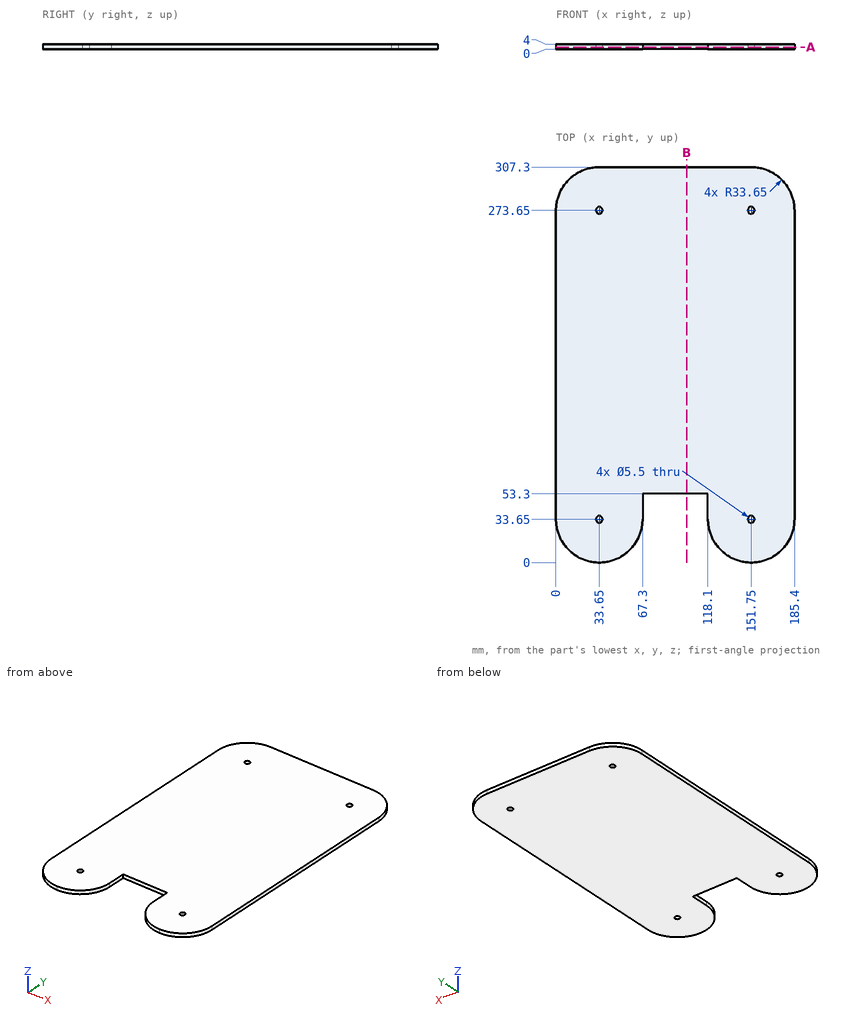
Verification items for this drawing (mm, ordinates from the low corner). Give positions to 0.01 mm unless a question says otherwise; leave off trailing zeros. Write each loop counter-clockwise with the first axis right and the second up, starting at its lowest first coordinate (ties: lowest second). Pieces come first, ordered by that corner, then holes.
1) Gauge pin test, flat ends, axial feed: pin 1 (1 mm diameter, centred on x = 28.5, z = 1.5, fed in from -Y); pin 2 (2 mm diameter, centred on y = 47.5, z = 2.5, fed in from -X); pin 3 (1 mm diameter, centred on x = 141.5, z = 2.5, fed in from -Y). Record the tip position at first contact, or that the pin passes through.
2) Section check A-A, the plane z = 1.65. Record the boundary of the cut face in (x, y), and give its area (3 significant figures).
3) Section check B-B, the plane x = 101.5. Record the boundary of the cut face in (y, z).
4) Material ranges on L1, parallel to Y at x = 151.75, z = 2.65; L2, parallel to X at y = 20, z = 3.5; L3, parallel to X at y = 21, z = 2, recorded low to high.
Computed:
1. pin 1: stops at y = 0.32
1. pin 2: stops at x = 0
1. pin 3: stops at y = 1.44
2. outline: (0, 33.65) arc R33.65 ccw to (67.3, 33.65) - (67.3, 53.3) - (118.1, 53.3) - (118.1, 33.65) arc R33.65 ccw to (185.4, 33.65) - (185.4, 273.65) arc R33.65 ccw to (151.75, 307.3) - (33.65, 307.3) arc R33.65 ccw to (0, 273.65) - close; hole circle Ø5.5 at (33.65, 33.65); hole circle Ø5.5 at (33.65, 273.65); hole circle Ø5.5 at (151.75, 33.65); hole circle Ø5.5 at (151.75, 273.65)
2. area: 52,700 mm2
3. outline: (53.3, 0) - (307.3, 0) - (307.3, 4) - (53.3, 4) - close
4. L1: y = 0 to 30.9, 36.4 to 270.9, 276.4 to 307.3
4. L2: x = 2.89 to 64.41, 120.99 to 182.51
4. L3: x = 2.47 to 64.83, 120.57 to 182.93
